from build123d import *

# Parameters (mm, degrees)
F0_W     = 67.1
F0_H     = 15.54066
F1_DEPTH = 25
F2_R     = 4.345584
F3_W     = 13.058827
F3_H     = 3
F4_DEPTH = 13
F5_W     = 17.786888
F5_H     = 3.586066
F6_DEPTH = 12.5


with BuildPart() as f1:
    # F0 (on Front) → F1 (new body)
    with BuildSketch(Plane.XZ):
        with Locations((3.872952, -1.860657)):
            Rectangle(F0_W, F0_H)
    extrude(amount=F1_DEPTH)

    # F2
    f2_edges = [f1.edges().sort_by_distance(p)[0] for p in [
        (37.422952, 0, -1.860657),
        (-29.677048, 0, -1.860657),
        (37.422952, -25, -1.860657),
        (-29.677048, -25, -1.860657),
    ]]
    fillet(f2_edges, radius=F2_R)

    # F3 (on face) → F4 (join)
    with BuildSketch(Plane.XZ.offset(25)):
        with Locations((3.352943, 0)):
            Rectangle(F3_W, F3_H)
    extrude(amount=F4_DEPTH)

    # F5 (on face) → F6 (cut, symmetric)
    with BuildSketch(Plane(origin=(0, 0, 0), x_dir=(-1, 0, 0), z_dir=(0, 1, 0))):
        with Locations((-2.295081, -1.793033)):
            Rectangle(F5_W, F5_H)
    extrude(amount=F6_DEPTH, both=True, mode=Mode.SUBTRACT)


solid = f1.part
Work out the finished part from the listing and answer in its coordinate system (mm). A direction names the side the tool comes from. Give positions to 0.01 mm unless a question says otherwise; leave off trailing zeros. Write each loop counter-clockwise with the first axis right and the second up, starting at its lowest first coordinate (ties: lowest second). Pieces come first, ordered by that corner, then holes.
Q1. The part is cut by section C-C on x = -9. Give the vertices of the cut face in (y, z), and give its area (3 significant figures).
Answer:
outline: (-25, -9.63) - (0, -9.63) - (0, 5.91) - (-25, 5.91) - close
area: 389 mm2
Q2. Straight lines are drawn through the part: L1, parallel to X at y = -8.5, z = -0.75; L2, parallel to Y at x = -9.5, z = -7.5; L3, parallel to Y at x = 6, z = -1.25. For each, find the intervals that lie inside material, in ascending order.
Answer:
L1: x = -29.68 to -6.6, 11.19 to 37.42
L2: y = -25 to 0
L3: y = -38 to -12.5
Q3. The part is cut by section B-B on z = -2.75. Give the vertices of the cut face in (x, y), and give its area (3 significant figures).
Answer:
outline: (-29.68, -20.65) arc R4.35 ccw to (-25.33, -25) - (33.08, -25) arc R4.35 ccw to (37.42, -20.65) - (37.42, -4.35) arc R4.35 ccw to (33.08, 0) - (11.19, 0) - (11.19, -12.5) - (-6.6, -12.5) - (-6.6, 0) - (-25.33, 0) arc R4.35 ccw to (-29.68, -4.35) - close
area: 1,440 mm2
Q4. Given pin 1 (5 mm diameter, centred on x = 15, z = -3, fed in from -Y); pin 2 (0.9 mm diameter, centred on y = -29, z = 0.5, fed in from +X); pin 3 (6 mm diameter, centred on y = -25, z = -5.5, fed in from +X), each flat-ended and moving along its own axis, determine where each tip first touches the part or whether it passes through.
Answer:
pin 1: stops at y = -25
pin 2: stops at x = 9.88
pin 3: stops at x = 37.21
Q5. For a pull along X with two mould halves and no side action, classify faces 5 (the face through (3, -31, 1.5)), 6 (the face through (2, -6, 0)), 7 (the face through (36.184, -23.693, -1.752)) as released by +X, released by -X, zero draft, split by the parting line, or undercut.
Answer:
face 5: zero draft
face 6: undercut
face 7: released by +X
Q6. The part is cut by section D-D on z = 3. Give the vertices of the cut face in (x, y), and give its area (3 significant figures).
Answer:
outline: (-29.68, -20.65) arc R4.35 ccw to (-25.33, -25) - (33.08, -25) arc R4.35 ccw to (37.42, -20.65) - (37.42, -4.35) arc R4.35 ccw to (33.08, 0) - (-25.33, 0) arc R4.35 ccw to (-29.68, -4.35) - close
area: 1,660 mm2
Q7. A tool of negligible diameter and unlimited length cuts with its end or side. For faces 1 (the face through (-29.677, -12, -2)), 2 (the face through (2, -6, -3.586)), 3 (the face through (-3.176, -31, 0)), 4 (the face through (3, -31, -1.5)), from which of +Z, -Z, +X, -X, +Y, -Y can it reach the whole face along a straight path? Write none if from no direction.
Answer:
face 1: +Z, -Z, -X, +Y, -Y
face 2: +Y
face 3: +Z, -Z, -X, -Y
face 4: -Z, +X, -X, -Y
Q8. The part is cut by section A-A on y = -6.5. Give the vertices of the cut face in (x, z).
Answer:
outline: (-29.68, -9.63) - (37.42, -9.63) - (37.42, 5.91) - (-29.68, 5.91) - close; hole (-6.6, -3.59) - (11.19, -3.59) - (11.19, 0) - (-6.6, 0) - close
